Work out the finished part from the listing and answer in its coordinate system (mm). Face numbers are marked on the shaded views. A direction names the side the tool comes from. Coordinates: 2 decimals unless noted, no trailing zeros. Order: outer loops, then holes, each group sorted by start corner. A loop starts at its lowest first (then second) coordinate and runs counter-clockwise, first axis right, second up. Notation, with made-up numbers: (26.25, 72) -> (34.25, 72) arc R23 cw to (34.25, 104) -> close; hole circle Ø9 at (77.5, 64.5). An arc over 180 degrees is marked (long way). Answer as CSV lines item,"result". Start each with the question number.
Item 1: For a pull along X with two mould halves and no side action, classify the marked faces 1, 2 and 3 as pulls with the +X half, pulls with the -X half, needs draft (parallel to the pull), parting line crosses it, or undercut.
Item 2: Section D-D (y = -24.5) is taken. Write down the section's boundary in (x, z).
Item 3: Which of the six approach directions +Z, -Z, +X, -X, +Y, -Y give full straight-line access (tool end or side, diameter ignored) to the marked faces 4 and 5?
Item 4: Section C-C (x = 17.5) is taken. Write down the section's boundary in (y, z).
Item 5: Straight lines are drawn through the part: L1, parallel to X at y = 1, z = 2.75 (3 decimals); L2, parallel to Y at x = -2, z = 2.1; L3, parallel to Y at x = 3, z = 1. For each, find the intervals that lie inside material, in ascending order.
Item 6: Each of these flat-tipped pins is pushed along its axis until it touches: pin 1 Ø1.5 at (x, z) = (1, 2.5) entering from +Y; pin 2 Ø1.5 at (x, z) = (-2, 1) entering from -Y; pin 3 Ø2 at (y, z) = (20.5, 3.5) entering from -X. Where does it stop, or does it pass through?
Item 7: Section A-A (z = 3.4) is taken. Count the separate pieces of the cut face and the enclosed holes in it, then the cut area to 3 significant figures.
Item 8: Section B-B (y = 32) is taken. Write down the section's boundary in (x, z), then the cut area to 3 significant figures.
```python
from build123d import *

# Parameters (mm, degrees)
SKETCH1_R           = 40
BOSS_EXTRUDE1_DEPTH = 5
CUT_EXTRUDE3_START  = -10
CUT_EXTRUDE3_DEPTH  = 10
FILLET1_R           = 30
FILLET2_R           = 25
SKETCH14_W          = 7.05
SKETCH14_H          = 5.05
CUT_EXTRUDE4_DEPTH  = 10
CUT_EXTRUDE5_START  = -1
CUT_EXTRUDE5_DEPTH  = 1


# Read off the part's stored shape, not the designer's step: Cut-Extrude5
with BuildPart() as part:
    # Sketch1 → Boss-Extrude1 (new body)
    with BuildSketch(Plane.XY):
        Circle(SKETCH1_R)
    extrude(amount=BOSS_EXTRUDE1_DEPTH)

    # Sketch10 → Cut-Extrude3 (cut)
    with BuildSketch(Plane.XY.offset(5).offset(CUT_EXTRUDE3_START)):
        with BuildLine():
            Line((-30, 26.457513111), (-30, -26.457513111))
            ThreePointArc((-30, -26.457513111), (-40, 0), (-30, 26.457513111))
        make_face()
        with BuildLine():
            Line((30, 26.457513111), (30, -26.457513111))
            ThreePointArc((30, -26.457513111), (40, 0), (30, 26.457513111))
        make_face()
    extrude(amount=CUT_EXTRUDE3_DEPTH, mode=Mode.SUBTRACT)

    # Fillet1
    fillet1_edges = [part.edges().sort_by_distance(p)[0] for p in [
        (-30, 26.457513111, 2.5),
        (30, 26.457513111, 2.5),
    ]]
    fillet(fillet1_edges, radius=FILLET1_R - 0.0001)  # a hair under: the kernel refuses the full size

    # Fillet2
    fillet2_edges = [part.edges().sort_by_distance(p)[0] for p in [
        (-30, -26.457513111, 2.5),
        (30, -26.457513111, 2.5),
    ]]
    fillet(fillet2_edges, radius=FILLET2_R)

    # Sketch14 → Cut-Extrude4 (cut)
    with BuildSketch(Plane.XY.offset(5)):
        with Locations((0, 1.975)):
            Rectangle(SKETCH14_W, SKETCH14_H)
        with Locations((0, -18.075)):
            Rectangle(SKETCH14_W, SKETCH14_H)
    extrude(amount=-CUT_EXTRUDE4_DEPTH, mode=Mode.SUBTRACT)

    # Cut-Extrude5 outline → Cut-Extrude5 (cut)
    with BuildSketch(Plane(origin=(0, 0, 0), x_dir=(-1, 0, 0), z_dir=(0, 0, -1)).offset(CUT_EXTRUDE5_START)):
        Polygon((15.056868042, 38), (14.160607491, 36.447631189), (9.918295379, 29.099731068), (14.248422398, 26.599731068), (18.36181188, 33.724330643), (20, 36.5617557), (20, 38), align=None)
    extrude(amount=CUT_EXTRUDE5_DEPTH, mode=Mode.SUBTRACT)


solid = part.part
```
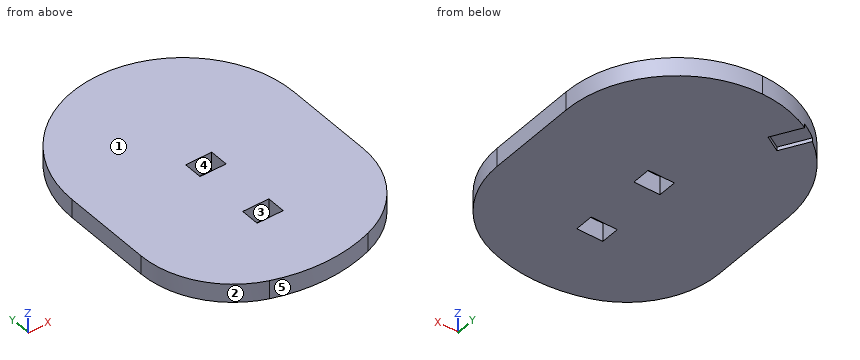
Checked values:
1,face 1,"needs draft"
1,face 2,"pulls with the -X half"
1,face 3,"undercut"
2,outline,"(-27.75, 0) -> (27.75, 0) -> (27.75, 5) -> (-27.75, 5) -> close"
3,face 4,"+Z, -Z"
3,face 5,"+Z, -Z, -Y"
4,outline,"(-35.79, 0) -> (34.37, 0) -> (34.37, 5) -> (-35.79, 5) -> close"
5,L1,"x = -30 to -3.525, 3.525 to 30"
5,L2,"y = -39.95 to -20.6, -15.55 to -0.55, 4.5 to 39.93"
5,L3,"y = -39.89 to -20.6, -15.55 to -0.55, 4.5 to 39.85"
6,pin 1,"stops at y = 40"
6,pin 2,"stops at y = -39.98"
6,pin 3,"stops at x = -28.46"
7,separate pieces,"1"
7,enclosed holes,"2"
7,area,"4,030 mm^2"
8,outline,"(-20.4, 0) -> (-17.37, 0) -> (-17.37, 1) -> (-11.59, 1) -> (-11.59, 0) -> (20.4, 0) -> (20.4, 5) -> (-20.4, 5) -> close"
8,area,"198 mm^2"
